from build123d import *

# Parameters (mm, degrees)
BOSS_EXTRUDE1_DEPTH   = 3
BOSS_EXTRUDE1_2_DEPTH = 3
SKETCH1_W             = 23.4
SKETCH1_H             = 29
SKETCH1_R             = 1
BOSS_EXTRUDE1_3_DEPTH = 3
FILLET1_R             = 2
SKETCH5_R             = 1.44
CUT_EXTRUDE3_DEPTH    = 10
CUT_EXTRUDE4_DEPTH    = 10
SKETCH8_R             = 1
CUT_EXTRUDE5_DEPTH    = 10
SKETCH9_R             = 3.026992654
BOSS_EXTRUDE3_DEPTH   = 3
SKETCH10_R            = 1.44
CUT_EXTRUDE6_DEPTH    = 3.5


with BuildPart() as part:
    # Sketch1 → Boss-Extrude1 (new body)
    with BuildSketch(Plane(origin=(0, 0, 0), x_dir=(1, 0, 0), z_dir=(0, 1, 0))):
        with BuildLine():
            add(Edge.make_bspline(
                [(19.180993887, -14.242526212), (19.80083761, -12.341053413), (17.899318471, -11.721194585), (17.279474749, -13.622667384), (16.659631026, -15.524140184), (18.561150164, -16.143999012), (19.180993887, -14.242526212)],
                knots=[0, 0, 0, 0, 0.5, 0.5, 0.5, 1, 1, 1, 1], degree=3, weights=[1, 0.333333333, 0.333333333, 1, 0.333333333, 0.333333333, 1]))
        make_face()
    extrude(amount=BOSS_EXTRUDE1_DEPTH)


with BuildPart() as body_2:
    # Sketch1 → Boss-Extrude1 2 (new body)
    with BuildSketch(Plane(origin=(0, 0, 0), x_dir=(1, 0, 0), z_dir=(0, 1, 0))):
        with BuildLine():
            add(Edge.make_bspline(
                [(22.488505608, -4.096188772), (23.108349331, -2.194715972), (21.206830193, -1.574857144), (20.58698647, -3.476329943), (19.967142747, -5.377802743), (21.868661885, -5.997661571), (22.488505608, -4.096188772)],
                knots=[0, 0, 0, 0, 0.5, 0.5, 0.5, 1, 1, 1, 1], degree=3, weights=[1, 0.333333333, 0.333333333, 1, 0.333333333, 0.333333333, 1]))
        make_face()
    extrude(amount=BOSS_EXTRUDE1_2_DEPTH)


with BuildPart() as body_3:
    # Sketch1 → Boss-Extrude1 3 (new body)
    with BuildSketch(Plane(origin=(0, 0, 0), x_dir=(1, 0, 0), z_dir=(0, 1, 0))):
        Rectangle(SKETCH1_W, SKETCH1_H)
        with Locations(Location((9, 8.9, 0), (0, 0, 270))):
            Circle(SKETCH1_R, mode=Mode.SUBTRACT)
        with Locations(Location((9, -8.5, 0), (0, 0, 90))):
            Circle(SKETCH1_R, mode=Mode.SUBTRACT)
        with Locations(Location((-9, -8.5, 0), (0, 0, 90))):
            Circle(SKETCH1_R, mode=Mode.SUBTRACT)
        with Locations(Location((1.7, -8.5, 0), (0, 0, 90))):
            Circle(SKETCH1_R, mode=Mode.SUBTRACT)
    extrude(amount=BOSS_EXTRUDE1_3_DEPTH)

    # Fillet1
    fillet1_edges = [body_3.edges().sort_by_distance(p)[0] for p in [
        (11.7, 1.5, 14.5),
        (-11.7, 1.5, 14.5),
        (-11.7, 1.5, -14.5),
        (11.7, 1.5, -14.5),
    ]]
    fillet(fillet1_edges, radius=FILLET1_R)

    # Sketch5 → Cut-Extrude3 (cut)
    with BuildSketch(Plane.XZ):
        with Locations(Location((-2.145634177, 3.61037734, 0), (0, 0, 270))):
            Circle(SKETCH5_R)
    extrude(amount=-CUT_EXTRUDE3_DEPTH, mode=Mode.SUBTRACT)

    # Sketch8 → Cut-Extrude5 (cut)
    with BuildSketch(Plane(origin=(0, 3, 0), x_dir=(1, 0, 0), z_dir=(0, 1, 0))):
        with Locations(Location((1.7, 8.9, 0), (0, 0, 270))):
            Circle(SKETCH8_R)
        with Locations(Location((-9, 8.9, 0), (0, 0, 270))):
            Circle(SKETCH8_R)
    extrude(amount=-CUT_EXTRUDE5_DEPTH, mode=Mode.SUBTRACT)

    # Sketch9 → Boss-Extrude3 (add)
    with BuildSketch(Plane(origin=(0, 3, 0), x_dir=(1, 0, 0), z_dir=(0, 1, 0))):
        with Locations((-2.145634177, -3.61037734)):
            Circle(SKETCH9_R)
    extrude(amount=-BOSS_EXTRUDE3_DEPTH)

    # Sketch10 → Cut-Extrude6 (cut)
    with BuildSketch(Plane(origin=(0, 3, 0), x_dir=(1, 0, 0), z_dir=(0, 1, 0))):
        with Locations(Location((-2.523984187, -0.0532018, 0), (0, 0, 270))):
            Circle(SKETCH10_R)
    extrude(amount=-CUT_EXTRUDE6_DEPTH, mode=Mode.SUBTRACT)


with BuildPart() as cut_extrude4_tool:
    # Sketch7 → Cut-Extrude4 (new body)
    with BuildSketch(Plane(origin=(0, 3, 0), x_dir=(1, 0, 0), z_dir=(0, 1, 0))):
        with BuildLine():
            add(Edge.make_bspline(
                [(19.180993887, -14.242526212), (19.80083761, -12.341053413), (17.899318471, -11.721194585), (17.279474749, -13.622667384), (16.659631026, -15.524140184), (18.561150164, -16.143999012), (19.180993887, -14.242526212)],
                knots=[0, 0, 0, 0, 0.5, 0.5, 0.5, 1, 1, 1, 1], degree=3, weights=[1, 0.333333333, 0.333333333, 1, 0.333333333, 0.333333333, 1]))
        make_face()
        with BuildLine():
            add(Edge.make_bspline(
                [(22.488505608, -4.096188772), (23.108349331, -2.194715972), (21.206830193, -1.574857144), (20.58698647, -3.476329943), (19.967142747, -5.377802743), (21.868661885, -5.997661571), (22.488505608, -4.096188772)],
                knots=[0, 0, 0, 0, 0.5, 0.5, 0.5, 1, 1, 1, 1], degree=3, weights=[1, 0.333333333, 0.333333333, 1, 0.333333333, 0.333333333, 1]))
        make_face()
    extrude(amount=-CUT_EXTRUDE4_DEPTH)


with BuildPart() as part_1:
    add(part.part)

    # Cut-Extrude4: cut by cut_extrude4_tool
    add(cut_extrude4_tool.part, mode=Mode.SUBTRACT)


with BuildPart() as body_2_1:
    add(body_2.part)

    # Cut-Extrude4: cut by cut_extrude4_tool
    add(cut_extrude4_tool.part, mode=Mode.SUBTRACT)


solid = body_3.part
Geometry: final body of the model. Coordinates: model frame, mm. Give positions to 0.01 mm unless a question says otherwise; leave off trailing zeros. Write each loop counter-clockwise with the first axis right and the second up, starting at its lowest first coordinate (ties: lowest second). Pieces come first, ordered by that corner, then holes. Notation, with made-up numbers: (26.25, 0.5) - (67.25, 0.5) arc R27 ccw to (67.25, 20.5) - close; hole circle Ø6 at (-27.5, 59.5). An arc over 180 degrees is marked (long way). Return JSON: item names as keys, results as strings. Group by question number.
1) Section B-B on z = -8.9. Return the cut outline in (x, y), plus the area to 3 significant figures.
2) Section C-C on y = 0.7. Return the cut outline in (x, z).
3) First-contact query: P1, Ø1.2, axis at x = -9, z = 8.5, coming from the +Y side; P2, Ø6, axis at x = 7.5, z = -5, coming from the -Y side. Flat tips, straight axial feed; report the tip coordinate or a pass-through.
4) Section D-D on x = -8.5. Return the cut outline in (y, z).
5) Line query: line 1 (X direction, y = 1.55, z = 8.5); line 2 (Z direction, x = 1.75, y = 1.1); line 3 (X direction, y = 0.45, z = -8.5). Output: solid intervals per line, ascending.
6) Section A-A on x = 9. Return the cut outline in (y, z).
7) Mould query, pull axis Z, two halves, no side actions, for faces 1 (the flat face through (0, 1, 14.5)), 2 (the flat face through (11.7, 1, 0)), 3 (the cylindrical face through (1.7, 1.5, 9.5)). Classes: released by +Z, released by -Z, zero draft, split by the parting line, or undercut.
Filled in:
{
 "1": {"outline": "(-11.7, 0) - (-10, 0) - (-10, 3) - (-11.7, 3) - close; (-8, 0) - (0.7, 0) - (0.7, 3) - (-8, 3) - close; (2.7, 0) - (8, 0) - (8, 3) - (2.7, 3) - close; (10, 0) - (11.7, 0) - (11.7, 3) - (10, 3) - close", "area": "52.2 mm^2"},
 "2": {"outline": "(-11.7, -12.5) arc R2 ccw to (-9.7, -14.5) - (9.7, -14.5) arc R2 ccw to (11.7, -12.5) - (11.7, 12.5) arc R2 ccw to (9.7, 14.5) - (-9.7, 14.5) arc R2 ccw to (-11.7, 12.5) - close; hole circle Ø2 at (-9, -8.9); hole circle Ø2 at (-9, 8.5); hole circle Ø2.88 at (-2.52, 0.05); hole circle Ø2 at (1.7, -8.9); hole circle Ø2 at (1.7, 8.5); hole circle Ø2 at (9, -8.9); hole circle Ø2 at (9, 8.5)"},
 "3": {"P1": "passes through", "P2": "stops at y = 0"},
 "4": {"outline": "(0, -14.5) - (3, -14.5) - (3, -9.77) - (0, -9.77) - close; (0, -8.03) - (3, -8.03) - (3, 7.63) - (0, 7.63) - close; (0, 9.37) - (3, 9.37) - (3, 14.5) - (0, 14.5) - close"},
 "5": {"line 1": "x = -11.7 to -10, -8 to 0.7, 2.7 to 8, 10 to 11.7", "line 2": "z = -14.5 to -9.9, -7.9 to 7.5, 9.5 to 14.5", "line 3": "x = -11.7 to -9.92, -8.08 to 0.78, 2.62 to 8.08, 9.92 to 11.7"},
 "6": {"outline": "(0, -14.5) - (3, -14.5) - (3, -9.9) - (0, -9.9) - close; (0, -7.9) - (3, -7.9) - (3, 7.5) - (0, 7.5) - close; (0, 9.5) - (3, 9.5) - (3, 14.5) - (0, 14.5) - close"},
 "7": {"face 1": "released by +Z", "face 2": "zero draft", "face 3": "undercut"}
}
